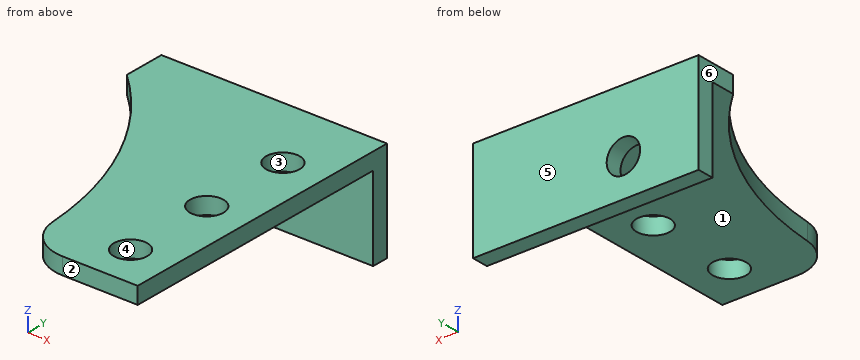
Autodesk Inventor part; units mm, degrees
ref_plane "YZ Plane" through (0, 0, 0) normal (1, 0, 0) x (0, 1, 0)
ref_plane "XZ Plane" through (0, 0, 0) normal (0, 1, 0) x (-1, 0, 0)
ref_plane "XY Plane" through (0, 0, 0) normal (0, 0, 1) x (1, 0, 0)
sketch "Sketch1" plane through (0, 0, 0) normal (1, 0, 0) x (0, 1, 0)
  line L0 (0, 0) -> (36, 0)
  line L1 (36, 0) -> (36, -12)
  line L2 (36, -12) -> (34, -12)
  line L3 (34, -12) -> (34, -2)
  line L4 (34, -2) -> (0, -2)
  line L5 (0, -2) -> (0, 0)
  dimension "d0" = 36
  dimension "d1" = 12
  dimension "d2" = 2
  dimension "d3" = 2
extrude "Extrusion1" add sketch "Sketch1" against normal blind 27
sketch "Sketch2" plane through (0, 36, 0) normal (0, 1, 0) x (1, 0, 0)
  circle A0 centre (-18, 7.5) radius 2
  line L0 (0, 0) -> (-27, 0)
  line L1 (0, 12) -> (0, 0)
  dimension "d6" = 4
  dimension "d7" = 7.5
  dimension "d8" = 18
extrude "Extrusion2" cut sketch "Sketch2" against normal blind 27
sketch "Sketch3" plane through (0, 0, 0) normal (0, 0, 1) x (1, 0, 0)
  line L0 (-27, 34) -> (-27, 0)
  line L1 (0, 36) -> (-27, 36)
  line L2 (-25.8683, 31) -> (-28.3872, 31) construction
  arc A0 (-13.9835, 4.5947) -> (-9, 0) centre (-9, 5) ccw
  line L3 (0, 0) -> (-27, 0)
  line L4 (0, 36) -> (0, 0)
  line L5 (-14, 4.4018) -> (-14, 0) construction
  circle A1 centre (-5, 27) radius 2
  circle A2 centre (-5, 16) radius 2
  circle A3 centre (-5, 5) radius 2
  line L6 (-27, 36) -> (0, 36)
  line L7 (0, 36) -> (0, 0)
  line L8 (0, 0) -> (-27, 0)
  line L9 (-27, 0) -> (-27, 36)
  arc A4 (-13.9835, 4.5947) -> (-27, 31) centre (-53.8519, 1.3525) ccw
  point P0 (-9, 0)
  dimension "d12" = 5
  dimension "d13" = 10
  dimension "d15" = 4
  dimension "d16" = 4
  dimension "d17" = 4
  dimension "d18" = 5
  dimension "d19" = 16
  dimension "d20" = 27
  dimension "d21" = 5
  dimension "d22" = 5
  dimension "d23" = 5
  dimension "d26" = 14
  dimension "d27" = 40
extrude "Extrusion3" cut sketch "Sketch3" against normal blind 27 contours A4 A0 L3 L0 | A1 | A2 | A3
Design review of the part built by this model. Coordinates are the model's own, in mm. Face numbers are marked on the shaded views. A direction names the side the tool comes from. Give positions to 0.01 mm unless a question says otherwise; leave off trailing zeros. Loops run counter-clockwise (first coordinate to the right, second up) from the corner with the lowest first, then second, coordinate; pieces in that order, holes last. Notation, with made-up numbers: M 40,12.5 L 93,12.5 A23 cw 93,32.5 Z; hole C -23.5,-8 d1. An arc over 180 degrees is marked long. One line per question, with ' | ' between items. Start each with the question number.
1. Add section D-D (x = -18). Write out the cut boundary in (y, z).
2. Add section C-C (y = 27). Write out the cut boundary in (x, z).
3. The part is to be moulded in two halves that separate along X. For the marked faces 3, 4, 5 and 6, say which applies: released by +X, released by -X, zero draft, split by the parting line, or undercut.
4. Insertion check: P1, Ø1.5, axis at x = -9.5, y = 13, coming from the +Z side; P2, Ø4.5, axis at x = -5, y = 16, coming from the -Z side; P3, Ø3, axis at x = -20, z = -5.5, coming from the -Y side. Each pin has a flat end and moves straight along its axis. Give the tip position at first contact, or say it passes through.
5. Add section A-A (z = -8.5). Write out the cut boundary in (x, y), plus the area to 3 significant figures.
6. For the marked faces 1 and 2, list the 3-axis set-ups (+Z, -Z, +X, -X, +Y, -Y) from which the entire face can be reached by the end or side of a thin tool; tool diameter is ignored.
7. Add section B-B (x = -5). Write out the cut boundary in (y, z), plus the area to 3 significant figures.
8. To check wall thickness, follow L1, parallel to Y at x = -5, z = -1.3; L2, parallel to Y at x = -2, z = -3.5; L3, parallel to X at y = 34.7, z = -7.5. State the ranges of each line that lie inside material, in increasing order.
Worked out:
1) outline: M 19.09,-2 L 34,-2 L 34,-5.5 L 36,-5.5 L 36,0 L 19.09,0 Z; M 34,-12 L 36,-12 L 36,-9.5 L 34,-9.5 Z
2) outline: M -23.16,-2 L -7,-2 L -7,0 L -23.16,0 Z; M -3,-2 L 0,-2 L 0,0 L -3,0 Z
3) face 3: undercut | face 4: undercut | face 5: zero draft | face 6: released by -X
4) P1: stops at z = 0 | P2: stops at z = -2 | P3: stops at y = 34
5) outline: M -27,34 L -19.73,34 L -19.73,36 L -27,36 Z; M -16.27,34 L 0,34 L 0,36 L -16.27,36 Z | area: 47.1 mm²
6) face 1: -Z, +X, -X, -Y | face 2: +Z, -Z, +X, -X, -Y
7) outline: M 0,-2 L 3,-2 L 3,0 L 0,0 Z; M 7,-2 L 14,-2 L 14,0 L 7,0 Z; M 18,-2 L 25,-2 L 25,0 L 18,0 Z; M 29,-2 L 34,-2 L 34,-12 L 36,-12 L 36,0 L 29,0 Z | area: 68.0 mm²
8) L1: y = 0 to 3, 7 to 14, 18 to 25, 29 to 36 | L2: y = 34 to 36 | L3: x = -27 to -20, -16 to 0
